Autodesk Inventor part; units mm, degrees
ref_plane "YZ Plane" through (0, 0, 0) normal (1, 0, 0) x (0, 1, 0)
ref_plane "XZ Plane" through (0, 0, 0) normal (0, 1, 0) x (-1, 0, 0)
ref_plane "XY Plane" through (0, 0, 0) normal (0, 0, 1) x (1, 0, 0)
sketch "Эскиз1" plane through (0, 0, 0) normal (0, 1, 0) x (-1, 0, 0)
  circle A0 centre (0, 0) radius 3.5
  dimension "d0" = 7
extrude "Выдавливание1" add sketch "Эскиз1" along normal blind 60
sketch "Эскиз3" plane through (0, 0, 0) normal (1, 0, 0) x (0, 1, 0)
  line L0 (0, 0) -> (0, -25)
  line L1 (0, -25) -> (-11.8591, -36.8591)
  line L2 (-11.8591, -36.8591) -> (-36.8591, -36.8591)
  line L3 (-36.8591, -32.8591) -> (-13.516, -32.8591)
  line L4 (-13.516, -32.8591) -> (-4, -23.3431)
  line L5 (-4, -23.3431) -> (-4, 0)
  line L6 (-36.8591, -32.8591) -> (-36.8591, -36.8591)
  line L7 (0, 0) -> (-15.7359, 0) construction
  line L8 (0, 0) -> (0, 25)
  line L9 (0, 25) -> (-11.8591, 36.8591)
  line L10 (-11.8591, 36.8591) -> (-36.8591, 36.8591)
  line L11 (-36.8591, 32.8591) -> (-13.516, 32.8591)
  line L12 (-13.516, 32.8591) -> (-4, 23.3431)
  line L13 (-4, 23.3431) -> (-4, 0)
  line L14 (-36.8591, 32.8591) -> (-36.8591, 36.8591)
  dimension "d7" = 25
  dimension "d8" = 45
  dimension "d9" = 25
  dimension "d10" = 4
extrude "Выдавливание3" add sketch "Эскиз3" along normal mid plane 7
sketch "Эскиз4" plane through (3.5, -11.8591, -36.8591) normal (0, 0, -1) x (-1, 0, 0)
  line L0 (7, -25) -> (0, -25)
  circle A0 centre (3.5, -25) radius 7.5
  point P0 (3.5, 11.8591)
  dimension "d13" = 15
extrude "Выдавливание4" add sketch "Эскиз4" against normal blind 5
mirror "Зеркальное отражение1" about plane through (0, 0, 0) normal (0, 0, 1) of "Выдавливание4"
sketch "Эскиз6" plane through (-3.5, -11.8591, 36.8591) normal (0, 0, 1) x (1, 0, 0)
  circle A0 centre (3.5, -25) radius 7.5
  circle A1 centre (3.5, -25) radius 3.5
  point P0 (3.5, 11.8591)
  dimension "d16" = 7
extrude "Выдавливание5" cut sketch "Эскиз6" against normal through all contours A1
properties part number "Макет_рамки" material "Алюминий 6061"
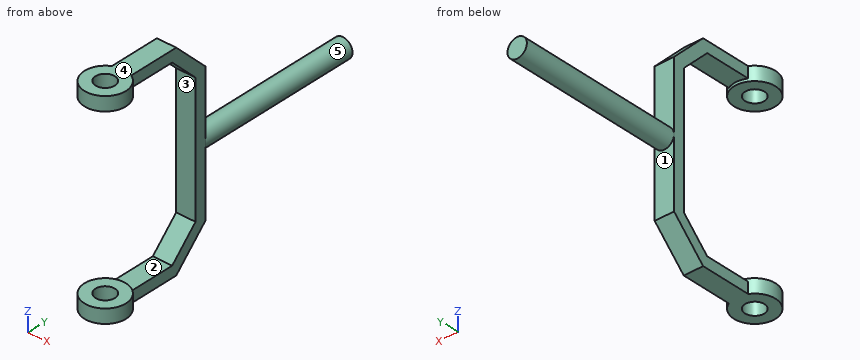
Build history of the part. All positions in model axes, mm. Face numbers are marked on the shaded views. A direction names the side the tool comes from. Give positions to 0.01 mm unless a question says otherwise; leave off trailing zeros. Write each loop counter-clockwise with the first axis right and the second up, starting at its lowest first coordinate (ties: lowest second). Pieces come first, ordered by that corner, then holes. Notation, with made-up numbers: (1, -33) - (36, -33) arc R31 cw to (36, -5) - close; hole circle Ø3 at (-19, 60.25). An arc over 180 degrees is marked (long way). Use one line per item in the form item = value. Start each with the question number.
1. 3-axis set-ups, long thin cutter, end or side, ignore diameter. For the marked faces 4 and 5: which of +Z, -Z, +X, -X, +Y, -Y reach the whole face in a straight line?
2. Band-saw the part on C-C on z = -13.5. Write the cut outline in (x, y).
3. Two-plate mould, pull along Y, no slides. Class the marked faces 1, 2 and 3: released by +Y, released by -Y, zero draft, split by the parting line, or undercut.
4. Probe line 1 (Y direction, x = -1, z = 8.5); line 2 (Y direction, x = 0, z = -34); line 3 (Y direction, x = 0, z = 34.3). List the from-to ranges inside material, lowest first. Write a range as [from, to].
5. Band-saw the part on D-D on y = 1.5. Write the cut outline in (x, z).
6. Band-saw the part on A-A on x = 0. Write the cut outline in (y, z), plus the area to 3 significant figures.
7. Band-saw the part on B-B on y = -16.5. Write the cut outline in (x, z), plus the area to 3 significant figures.
8. Drop flat-ended pins along their axis: pin 1 Ø8 at (x, z) = (4, -17.5) entering from -Y; pin 2 Ø15 at (y, z) = (-8, 13) entering from +X; pin 3 Ø5 at (y, z) = (39, 6.5) entering from -X; pin 4 Ø5.5 at (x, z) = (1, -8.5) entering from +Y. Give the stop position or say it passes through.
Conclusion:
q1.face_4 = +Z, +X, -X, +Y, -Y
q1.face_5 = +Y
q2.outline = (-3.5, -4) - (3.5, -4) - (3.5, 0) - (-3.5, 0) - close
q3.face_1 = released by +Y
q3.face_2 = undercut
q3.face_3 = released by -Y
q4.line_1 = [-4, 0]
q4.line_2 = [-44.36, -40.36], [-33.36, -9]
q4.line_3 = [-44.36, -40.36], [-33.36, -9.3]
q5.outline = circle Ø7 at (0, 0)
q6.outline = (-44.36, -36.86) - (-40.36, -36.86) - (-40.36, -31.86) - (-44.36, -31.86) - close; (-44.36, 31.86) - (-40.36, 31.86) - (-40.36, 36.86) - (-44.36, 36.86) - close; (-33.36, -36.86) - (-11.86, -36.86) - (0, -25) - (0, -3.5) - (60, -3.5) - (60, 3.5) - (0, 3.5) - (0, 25) - (-11.86, 36.86) - (-33.36, 36.86) - (-33.36, 31.86) - (-29.36, 31.86) - (-29.36, 32.86) - (-13.52, 32.86) - (-4, 23.34) - (-4, -23.34) - (-13.52, -32.86) - (-29.36, -32.86) - (-29.36, -31.86) - (-33.36, -31.86) - close
q6.area = 948 mm²
q7.outline = (-3.5, -36.86) - (3.5, -36.86) - (3.5, -32.86) - (-3.5, -32.86) - close; (-3.5, 32.86) - (3.5, 32.86) - (3.5, 36.86) - (-3.5, 36.86) - close
q7.area = 56.0 mm²
q8.pin_1 = -4
q8.pin_2 = 3.5
q8.pin_3 = through
q8.pin_4 = 0
